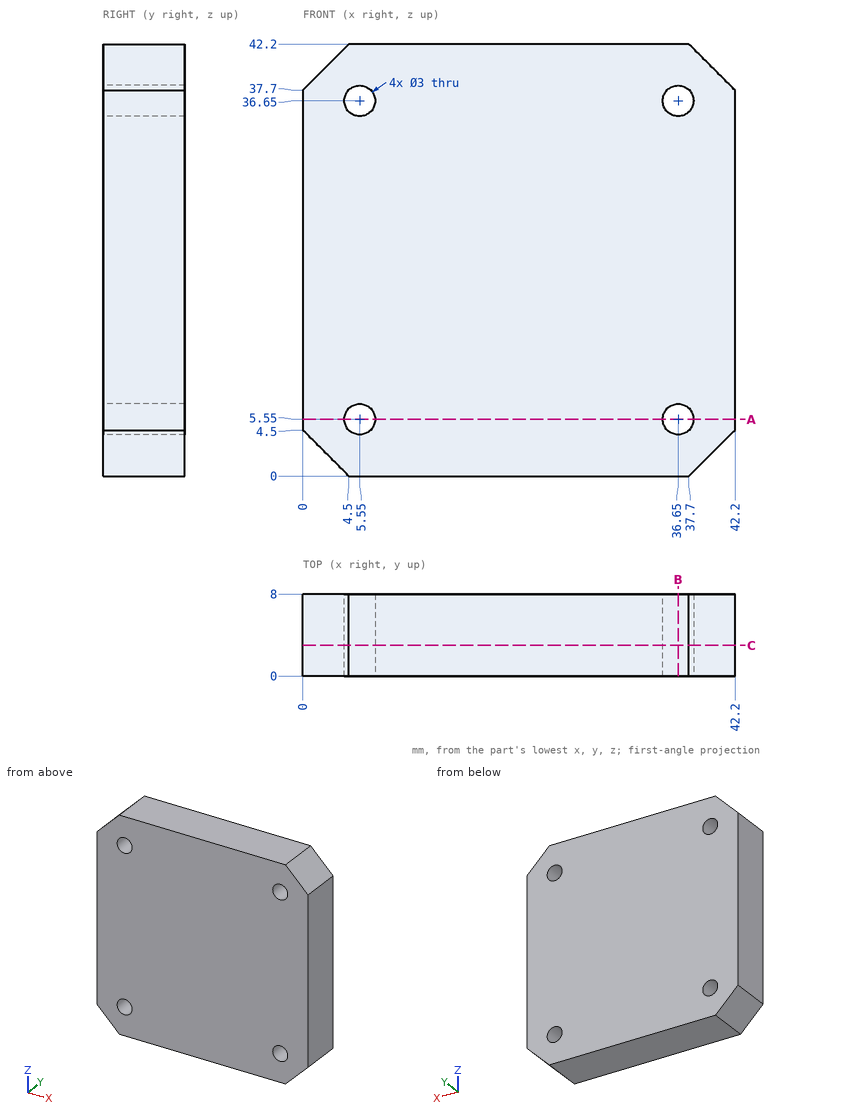
Geometry check sheet. Reference: drawing and pictorial views, mm from the part's lowest x, y, z. Coordinates: 2 decimals unless noted, no trailing zeros. Order: outer loops, then holes, each group sorted by start corner. A loop starts at its lowest first (then second) coordinate and runs counter-clockwise, first axis right, second up.
Item 1: Section check A-A (z = 5.55). Enter the section's corners in (x, y), plus the area to 3 significant figures.
Item 2: Section check C-C (y = 3). Enter the section's corners in (x, z).
Item 3: Section check B-B (x = 36.65). Enter the section's corners in (y, z).
Item 4: Scan lines: line 1 along Z through (x, y) = (5.55, 2.75); line 2 along Z through (x, y) = (39.5, 6). Record each from-to range of solid material in increasing order.
Check sheet entries:
1. outline: (0, 0) - (4.05, 0) - (4.05, 8) - (0, 8) - close; (7.05, 0) - (35.15, 0) - (35.15, 8) - (7.05, 8) - close; (38.15, 0) - (42.2, 0) - (42.2, 8) - (38.15, 8) - close
1. area: 290 mm2
2. outline: (0, 4.5) - (4.5, 0) - (37.7, 0) - (42.2, 4.5) - (42.2, 37.7) - (37.7, 42.2) - (4.5, 42.2) - (0, 37.7) - close; hole circle Ø3 at (5.55, 5.55); hole circle Ø3 at (5.55, 36.65); hole circle Ø3 at (36.65, 5.55); hole circle Ø3 at (36.65, 36.65)
3. outline: (0, 0) - (8, 0) - (8, 4.05) - (0, 4.05) - close; (0, 7.05) - (8, 7.05) - (8, 35.15) - (0, 35.15) - close; (0, 38.15) - (8, 38.15) - (8, 42.2) - (0, 42.2) - close
4. line 1: z = 0 to 4.05, 7.05 to 35.15, 38.15 to 42.2
4. line 2: z = 1.8 to 40.4
